from build123d import *

# Parameters (mm, degrees)
SKETCH1_W                = 47
SKETCH1_H                = 39.4
BOSS_EXTRUDE1_DEPTH      = 50
SKETCH3_W                = 10.5
SKETCH3_H                = 30
CUT_EXTRUDE1_DEPTH       = 50
SKETCH19_R               = 5
CUT_EXTRUDE6_DEPTH       = 68.857276692
M5_CLEARANCE_HOLE1_D     = 5.5
M5_CLEARANCE_HOLE1_DEPTH = 6
SKETCH25_R               = 7.5
CUT_EXTRUDE7_DEPTH       = 28
CUT_EXTRUDE8_DEPTH       = 28
SKETCH27_W               = 26
SKETCH27_H               = 16
CUT_EXTRUDE9_DEPTH       = 28
CUT_EXTRUDE10_REACH      = 69.857
SKETCH28_R               = 1.7
BOSS_EXTRUDE2_DEPTH      = 26
SKETCH30_W               = 16
SKETCH30_H               = 41.736735488
CUT_EXTRUDE11_DEPTH      = 28
BOSS_EXTRUDE3_DEPTH      = 11.4
CHAMFER1_SIZE            = 2


with BuildPart() as part:
    # Sketch1 → Boss-Extrude1 (new body)
    with BuildSketch(Plane.XY):
        Rectangle(SKETCH1_W, SKETCH1_H)
    extrude(amount=BOSS_EXTRUDE1_DEPTH)

    # Sketch3 → Cut-Extrude1 (cut)
    with BuildSketch(Plane(origin=(0, 19.7, 0), x_dir=(1, 0, 0), z_dir=(0, 1, 0))):
        with Locations((18.25, -21)):
            Rectangle(SKETCH3_W, SKETCH3_H)
        with Locations((-18.25, -21)):
            Rectangle(SKETCH3_W, SKETCH3_H)
    extrude(amount=-CUT_EXTRUDE1_DEPTH, mode=Mode.SUBTRACT)

    # Sketch19 → Cut-Extrude6 (cut, through all)
    with BuildSketch(Plane.XZ.offset(19.7)):
        with Locations(Location((0, 13, 0), (0, 0, 270))):
            Circle(SKETCH19_R)
    extrude(amount=-CUT_EXTRUDE6_DEPTH, mode=Mode.SUBTRACT)

    # M5 Clearance Hole1
    with Locations(Plane(origin=(0, 0, 0), x_dir=(-1, 0, 0), z_dir=(0, 0, -1))):
        with Locations((-19, -15), (-19, 15), (19, 15), (19, -15)):
            Hole(M5_CLEARANCE_HOLE1_D / 2, depth=M5_CLEARANCE_HOLE1_DEPTH)

    # Sketch25 → Cut-Extrude7 (cut)
    with BuildSketch(Plane(origin=(0, 19.7, 0), x_dir=(1, 0, 0), z_dir=(0, 1, 0))):
        with Locations(Location((0, -13, 0), (0, 0, 270))):
            Circle(SKETCH25_R)
    extrude(amount=-CUT_EXTRUDE7_DEPTH, mode=Mode.SUBTRACT)

    # Sketch26 → Cut-Extrude8 (cut)
    with BuildSketch(Plane(origin=(0, 19.7, 0), x_dir=(1, 0, 0), z_dir=(0, 1, 0))):
        Polygon((13, -6), (13, -36), (23.5, -36), (23.5, -50), (-23.5, -50), (-23.5, -36), (-13, -36), (-13, -6), align=None)
    extrude(amount=-CUT_EXTRUDE8_DEPTH, mode=Mode.SUBTRACT)

    # Sketch27 → Cut-Extrude9 (cut)
    with BuildSketch(Plane.XY.offset(6)):
        with Locations((0, -0.3)):
            Rectangle(SKETCH27_W, SKETCH27_H)
    extrude(amount=-CUT_EXTRUDE9_DEPTH, mode=Mode.SUBTRACT)

    # Sketch28 → Cut-Extrude10 (cut, up to next)
    with BuildSketch(Plane.XZ.offset(19.7), mode=Mode.PRIVATE) as cut_extrude10_sk1:
        with Locations(Location((0, 21, 0), (0, 0, 270))):
            Circle(SKETCH28_R)
    cut_extrude10_tool1 = extrude(cut_extrude10_sk1.sketch, amount=-CUT_EXTRUDE10_REACH, mode=Mode.PRIVATE) & part.part
    # Sketch28 → Cut-Extrude10 (cut, up to next)
    with BuildSketch(Plane.XZ.offset(19.7), mode=Mode.PRIVATE) as cut_extrude10_sk2:
        with Locations(Location((8, 13, 0), (0, 0, 270))):
            Circle(SKETCH28_R)
    cut_extrude10_tool2 = extrude(cut_extrude10_sk2.sketch, amount=-CUT_EXTRUDE10_REACH, mode=Mode.PRIVATE) & part.part
    # Sketch28 → Cut-Extrude10 (cut, up to next)
    with BuildSketch(Plane.XZ.offset(19.7), mode=Mode.PRIVATE) as cut_extrude10_sk3:
        with Locations(Location((0, 5, 0), (0, 0, 270))):
            Circle(SKETCH28_R)
    cut_extrude10_tool3 = extrude(cut_extrude10_sk3.sketch, amount=-CUT_EXTRUDE10_REACH, mode=Mode.PRIVATE) & part.part
    # Sketch28 → Cut-Extrude10 (cut, up to next)
    with BuildSketch(Plane.XZ.offset(19.7), mode=Mode.PRIVATE) as cut_extrude10_sk4:
        with Locations(Location((-8, 13, 0), (0, 0, 270))):
            Circle(SKETCH28_R)
    cut_extrude10_tool4 = extrude(cut_extrude10_sk4.sketch, amount=-CUT_EXTRUDE10_REACH, mode=Mode.PRIVATE) & part.part
    # Sketch28 → Cut-Extrude10 (cut, up to next)
    with BuildSketch(Plane.XZ.offset(19.7), mode=Mode.PRIVATE) as cut_extrude10_sk5:
        with Locations(Location((-18.5, 45, 0), (0, 0, 270))):
            Circle(SKETCH28_R)
    cut_extrude10_tool5 = extrude(cut_extrude10_sk5.sketch, amount=-CUT_EXTRUDE10_REACH, mode=Mode.PRIVATE) & part.part
    # Sketch28 → Cut-Extrude10 (cut, up to next)
    with BuildSketch(Plane.XZ.offset(19.7), mode=Mode.PRIVATE) as cut_extrude10_sk6:
        with Locations(Location((18.5, 45, 0), (0, 0, 270))):
            Circle(SKETCH28_R)
    cut_extrude10_tool6 = extrude(cut_extrude10_sk6.sketch, amount=-CUT_EXTRUDE10_REACH, mode=Mode.PRIVATE) & part.part
    add(cut_extrude10_tool1.solids().sort_by_distance((0, -19.7, 21))[0], mode=Mode.SUBTRACT)
    add(cut_extrude10_tool2.solids().sort_by_distance((8, -19.7, 13))[0], mode=Mode.SUBTRACT)
    add(cut_extrude10_tool3.solids().sort_by_distance((0, -19.7, 5))[0], mode=Mode.SUBTRACT)
    add(cut_extrude10_tool4.solids().sort_by_distance((-8, -19.7, 13))[0], mode=Mode.SUBTRACT)
    add(cut_extrude10_tool5.solids().sort_by_distance((-18.5, -19.7, 45))[0], mode=Mode.SUBTRACT)
    add(cut_extrude10_tool6.solids().sort_by_distance((18.5, -19.7, 45))[0], mode=Mode.SUBTRACT)

    # Sketch29 → Boss-Extrude2 (add)
    with BuildSketch(Plane(origin=(13, 0, 0), x_dir=(0, 0, -1), z_dir=(1, 0, 0))):
        Polygon((-42.205748108, -8.3), (-30.205748108, -8.3), (-6, 9.919793382), (-6, 19.7), (-8.659491381, 19.7), align=None)
    extrude(amount=-BOSS_EXTRUDE2_DEPTH)

    # Sketch30 → Cut-Extrude11 (cut)
    with BuildSketch(Plane(origin=(0, 19.7, 0), x_dir=(1, 0, 0), z_dir=(0, 1, 0))):
        with Locations((0, -26.868367744)):
            Rectangle(SKETCH30_W, SKETCH30_H)
    extrude(amount=-CUT_EXTRUDE11_DEPTH, mode=Mode.SUBTRACT)

    # Sketch31 → Boss-Extrude3 (add)
    with BuildSketch(Plane.XZ.offset(19.7)):
        Polygon((-23.5, 36), (-13, 36), (-13, 27.846939537), align=None)
        Polygon((13, 36), (13, 27.846939537), (23.5, 36), align=None)
    extrude(amount=-BOSS_EXTRUDE3_DEPTH)

    # Chamfer1
    chamfer1_edges = [part.edges().sort_by_distance(p)[0] for p in [
        (23.5, -14, 50),
        (-23.5, -14, 50),
    ]]
    chamfer(chamfer1_edges, length=CHAMFER1_SIZE)


solid = part.part
Input: part model. Units: mm. Frame: model coordinates. A direction names the side the tool comes from. Give positions to 0.01 mm unless a question says otherwise; leave off trailing zeros. Loops run counter-clockwise (first coordinate to the right, second up) from the corner with the lowest first, then second, coordinate; pieces in that order, holes last. Notation, with made-up numbers: M -26,78.25 L 15,78.25 A19 ccw 15,82.25 Z; hole C 79.25,3.5 d1. An arc over 180 degrees is marked long. Use one line per item in the form item = value.
1. Section query B-B, the plane y = -15. Count the separate pieces of the cut face and the enclosed holes in it, and give its area (3 significant figures).
Numbers:
separate_pieces = 3
enclosed_holes = 7
area = 1,600 mm²
2. Section query C-C, the plane z = 13. Return the cut outline in (x, y).
Numbers:
outline = M -13,-19.7 L -9.7,-19.7 L -9.7,-8.3 L -13,-8.3 Z; M -13,4.65 L -8,4.65 L -8,16.08 L -13,16.08 Z; M -6.3,-19.7 L -5,-19.7 L -5,-8.3 L -6.3,-8.3 Z; M 5,-19.7 L 6.3,-19.7 L 6.3,-8.3 L 5,-8.3 Z; M 8,4.65 L 13,4.65 L 13,16.08 L 8,16.08 Z; M 9.7,-19.7 L 13,-19.7 L 13,-8.3 L 9.7,-8.3 Z
3. Line query: L1, parallel to X at y = -10, z = 13; L2, parallel to Z at x = -1, y = -16; L3, parallel to X at y = -11, z = 21. Output: solid intervals per line, ascending.
Numbers:
L1 = -13 to -9.7, -6.3 to -5, 5 to 6.3, 9.7 to 13
L2 = 0 to 3.63, 6.37 to 8.1, 17.9 to 19.63, 22.37 to 50
L3 = -13 to -1.7, 1.7 to 13
4. Section query A-A, the plane x = 4. Return the cut outline in (y, z).
Numbers:
outline = M -19.7,0 L -8.3,0 L -8.3,10 L -19.7,10 Z; M -19.7,16 L -8.3,16 L -8.3,50 L -19.7,50 Z; M 7.7,0 L 19.7,0 L 19.7,6 L 7.7,6 Z
5. Reachability of faces 1 (the face through (-13, 0, 3)), 2 (the face through (0, 13.8, 5.5)), 3 (the face through (-18.18, -14.08, 31.87)), 4 (the face through (18.18, -14.08, 31.87)) from +Z, -Z, +X, -X, +Y, -Y: full face, straight path, thin tool, end or side. Return the list, or none.
Numbers:
face_1 = -Z
face_2 = +Z, +Y
face_3 = -X, +Y, -Y
face_4 = +X, +Y, -Y
6. Section query D-D, the plane y = -7. Return the cut outline in (x, z).
Numbers:
outline = M -23.5,0 L -13,0 L -13,6 L -23.5,6 Z; M -13,28.48 L -8,28.48 L -8,40.65 L -13,40.65 Z; M 8,28.48 L 13,28.48 L 13,40.65 L 8,40.65 Z; M 13,0 L 23.5,0 L 23.5,6 L 13,6 Z
7. Pull-direction query (Z, two-part tool) for faces 5 (the face through (22.5, -14.1, 49)), 6 (the face through (18.642, 17.727, 3.042)), 7 (the face through (19.65, -14.08, 46.25)); classes: released by +Z, released by -Z, zero draft, split by the parting line, or undercut.
Numbers:
face_5 = released by +Z
face_6 = zero draft
face_7 = undercut
8. First-contact query: pin 1 (1 mm diameter, centred on x = 17, z = 36.5, fed in from +Y); pin 2 (3.5 mm diameter, centred on y = -11.5, z = 14.5, fed in from +X); pin 3 (7 mm diameter, centred on x = -19, y = 15, fed in from -Z); pin 4 (9 mm diameter, centred on x = 19, y = 15, fed in from +Z). Flat tips, straight axial feed; report the tip coordinate or a pass-through.
Numbers:
pin_1 = -8.3
pin_2 = 13
pin_3 = 0
pin_4 = 6
